Source: CAD feature listing. Evaluate the final solid. Frame: model axes, mm. Face numbers are marked on the shaded views. Coordinates: 2 decimals unless noted, no trailing zeros. Write each loop counter-clockwise with the first axis right and the second up, starting at its lowest first coordinate (ties: lowest second). Pieces come first, ordered by that corner, then holes. Notation, with made-up numbers: M 88,35 L 133,35 A11 cw 133,56 Z; hole C 53,-24.5 d2. An arc over 180 degrees is marked long. Write item = value, one per line. Start each with the question number.
1. Pull-direction query (X, two-part tool) for the marked faces 1, 2 and 3; classes: pulls with the +X half, pulls with the -X half, needs draft (parallel to the pull), parting line crosses it, or undercut.
2. Section query A-A (y = 0). Output: boundary loops of the cut face in (x, z), then the cut area to 3 significant figures.
3. Section query B-B (x = 37). Output: boundary loops of the cut face in (y, z).
4. Section query C-C (z = 71). Output: boundary loops of the cut face in (x, y).
5. Pin query (flat end, axial travel): pin 1 Ø1.5 at (x, z) = (-21.5, 86) entering from -Y; pin 2 Ø1.3 at (y, z) = (49.5, 74.5) entering from +X; pin 3 Ø0.8 at (y, z) = (-44, 36) entering from -X. Return the tip coordinate at first contact, or that it passes through.
6. Line query: line 1 along Y through (x, z) = (-42, 34.5); line 2 along Y through (x, z) = (-25.5, 91.5); line 3 along X through (y, z) = (37, 76). Output: solid intervals per line, ascending.
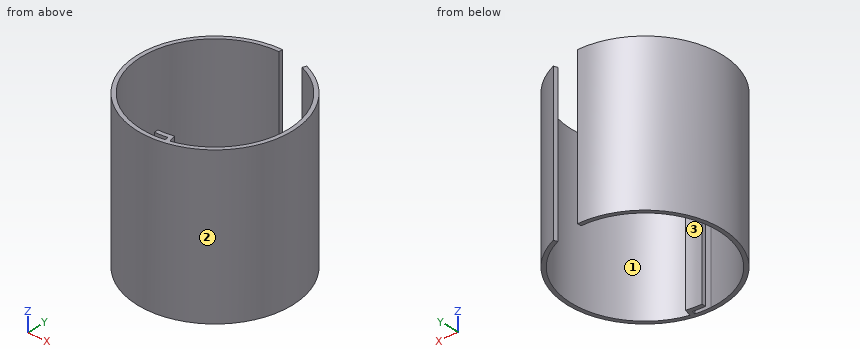
```python
from build123d import *

# Parameters (mm, degrees)
BOSS_EXTRUDE1_DEPTH = 101.6


with BuildPart() as part:
    # Sketch1 → Boss-Extrude1 (new body)
    with BuildSketch(Plane.XY):
        with BuildLine():
            Line((-1.27, 50.784122519), (-1.27, 48.24328658))
            ThreePointArc((-1.27, 48.24328658), (-48.255821464, -0.635054985), (0, -48.26))
            ThreePointArc((0, -48.26), (4.873264732, -48.013319932), (9.696710265, -47.275801527))
            Line((9.696710265, -47.275801527), (9.201166175, -44.859802346))
            ThreePointArc((9.201166175, -44.859802346), (5.255589984, -45.491121106), (1.27, -45.776090108))
            Line((1.27, -45.776090108), (1.27, -43.161319489))
            ThreePointArc((1.27, -43.161319489), (6.147836333, -42.740104216), (10.946634308, -41.769409827))
            Line((10.946634308, -41.769409827), (12.234473638, -46.683458042))
            ThreePointArc((12.234473638, -46.683458042), (48.208106465, -2.237425089), (16.505892117, 45.349565879))
            Line((16.505892117, 45.349565879), (17.374623281, 47.736385136))
            ThreePointArc((17.374623281, 47.736385136), (-8.195236332, -50.134599843), (-1.27, 50.784122519))
        make_face()
    extrude(amount=BOSS_EXTRUDE1_DEPTH)


solid = part.part
```
Results are:
q1.face_1 = undercut
q1.face_2 = parting line crosses it
q1.face_3 = undercut
q2.outline = M -50.8,0 L -48.26,0 L -48.26,101.6 L -50.8,101.6 Z; M 48.26,0 L 50.8,0 L 50.8,101.6 L 48.26,101.6 Z
q2.area = 516 mm^2
q3.outline = M -34.81,0 L -30.98,0 L -30.98,101.6 L -34.81,101.6 Z; M 30.98,0 L 34.81,0 L 34.81,101.6 L 30.98,101.6 Z
q4.outline = M -1.27,48.24 L -1.27,50.78 A50.8 ccw long 17.37,47.74 L 16.51,45.35 A48.26 cw 12.23,-46.68 L 10.95,-41.77 A43.18 cw 1.27,-43.16 L 1.27,-45.78 A45.79 ccw 9.2,-44.86 L 9.7,-47.28 A48.26 cw long Z
q5.pin_1 = -46.37
q5.pin_2 = -1.27
q5.pin_3 = -26.07
q6.line_1 = -28.58 to -23.77, 23.77 to 28.58
q6.line_2 = -43.94 to -40.97, 40.97 to 43.94
q6.line_3 = -34.81 to -30.98, 30.98 to 34.81
